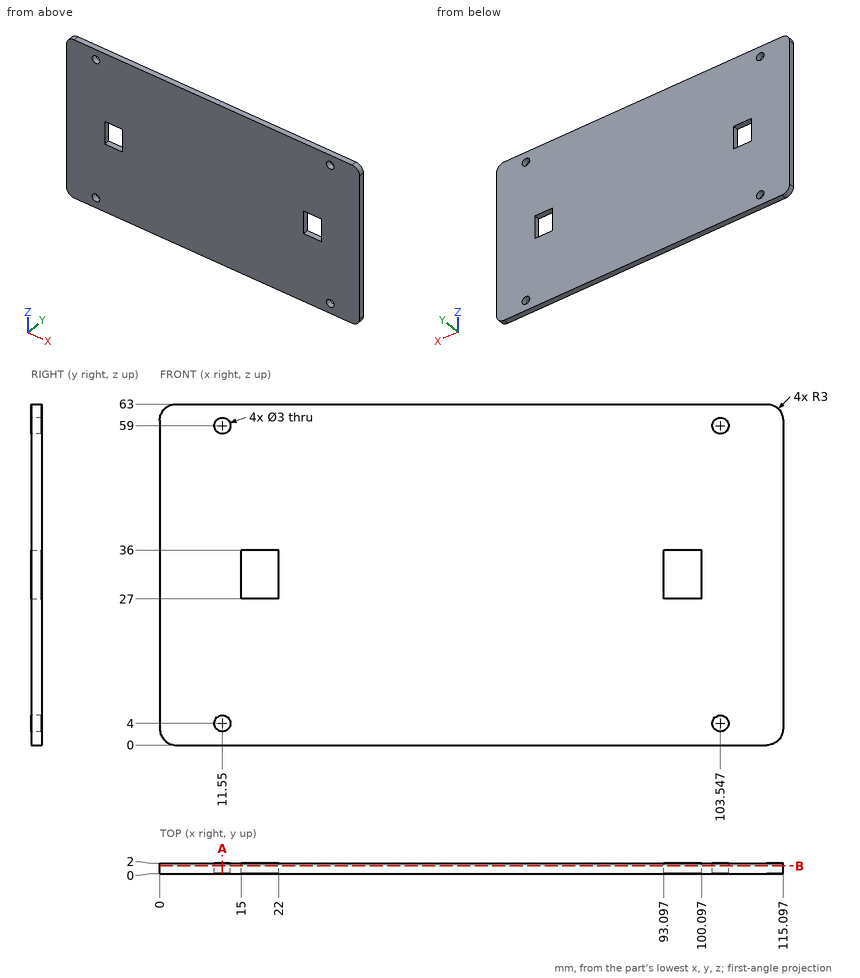
For this review, use the dimensioned drawing (mm, ordinates from the lowest corner) and the shaded views. Round coordinates to 2 decimals unless told otherwise and drop trailing zeros. Order: outer loops, then holes, each group sorted by start corner. A loop starts at its lowest first (then second) coordinate and runs counter-clockwise, first axis right, second up.
1) Consider section B-B (y = 1.5). State the section outline as (x, z) points.
The answers:
outline: (0, 3) arc R3 ccw to (3, 0) - (112.1, 0) arc R3 ccw to (115.1, 3) - (115.1, 60) arc R3 ccw to (112.1, 63) - (3, 63) arc R3 ccw to (0, 60) - close; hole circle Ø3 at (11.55, 4); hole circle Ø3 at (11.55, 59); hole (15, 27) - (22, 27) - (22, 36) - (15, 36) - close; hole (93.1, 27) - (100.1, 27) - (100.1, 36) - (93.1, 36) - close; hole circle Ø3 at (103.55, 4); hole circle Ø3 at (103.55, 59)
2) For L1, parallel to X at y = 1.6, z = 59; L2, parallel to X at y = 1.9, z = 27.5; L3, parallel to Z at x = 98, y = 1, list the stretches that pass through material, from the lowest coordinate up.
The answers:
L1: x = 0 to 10.05, 13.05 to 102.05, 105.05 to 115.1
L2: x = 0 to 15, 22 to 93.1, 100.1 to 115.1
L3: z = 0 to 27, 36 to 63
3) Clearance check with a flat-ended pin moving along its axis: pin 1 Ø2.5 at (x, z) = (103.55, 59) entering from -Y. State where the tip first meets the part, or that it passes through.
The answers:
pin 1: passes through
4) Consider section A-A (x = 11.55). State the section outline as (y, z) points, plus the area to 3 significant figures.
The answers:
outline: (0, 0) - (2, 0) - (2, 2.5) - (0, 2.5) - close; (0, 5.5) - (2, 5.5) - (2, 57.5) - (0, 57.5) - close; (0, 60.5) - (2, 60.5) - (2, 63) - (0, 63) - close
area: 114 mm2
